Part model, mm, in its own coordinate system. Face numbers are marked on the shaded views. A direction names the side the tool comes from. Round coordinates to 2 decimals unless told otherwise and drop trailing zeros. Write each loop counter-clockwise with the first axis right and the second up, starting at its lowest first coordinate (ties: lowest second). Pieces come first, ordered by that corner, then holes. Notation, with made-up numbers: M -33.75,-22.75 L 16.25,-22.75 A12 cw 16.25,-2.75 Z; hole C 83,-34.75 d8. An arc over 180 degrees is marked long. Use a Markdown table: item, result. Add a question column.
1) Two-plate mould, pull along X, no slides. Class the marked faces 1, 2 and 3: released by +X, released by -X, zero draft, split by the parting line, or undercut.
2) Slice it at C-C on z = 5.5. Write the cut outline in (x, y), plus the area to 3 significant figures.
3) Which spindle directions (+Z, -Z, +X, -X, +Y, -Y) get a long thin tool onto all of the face, cutting with end or side? Do the marked faces 4 and 5. Say none if no direction does.
4) Slice it at D-D on y = 10. Write the cut outline in (x, z).
5) Slice it at B-B on y = -14.5. Write the cut outline in (x, z).
6) Slice it at A-A on z = 1.5. Write the cut outline in (x, y).
7) Wall check: probe 1 along Y at (x, z) = (3.25, 6.25); probe 2 along X at (y, z) = (-10, 1.25); probe 3 along X at (y, z) = (14.5, 3.75). Give the ranges that are in metal, low to high.
8) Drop flat-ended pins along their axis: P1, Ø4, axis at x = 1, y = 15, coming from the -Z side; P2, Ø0.5, axis at x = 8, z = 7, coming from the -Y side; P3, Ø2.5, axis at x = 6, y = -11, coming from the -Z side. Give the stop position or say it passes through.
Solid Edge part; units mm, degrees
sketch "Sketch1" plane through (0, 0, 0) normal (0, 0, 1) x (1, 0, 0)
  line L0 (-4, -20) -> (4, -20)
  line L1 (4, -20) -> (4, 20)
  line L2 (4, 20) -> (-4, 20)
  line L3 (-4, 20) -> (-4, -20)
  dimension "D1" = 4
  dimension "D2" = 4
extrude "Protrusion1" add sketch "Sketch1" along normal blind 10
sketch "Sketch2" plane through (0, 0, 10) normal (0, 0, 1) x (0, 1, 0)
  line L0 (-15.5, -4) -> (-17.5, -7.5)
  line L1 (-17.5, -7.5) -> (-17.5, -9)
  line L2 (-17.5, -9) -> (-7.5, -9)
  line L3 (-7.5, -9) -> (-7.5, -7.5)
  line L4 (-7.5, -7.5) -> (-9.5, -4)
  line L5 (-15.5, -4) -> (-9.5, -4)
  dimension "D1" = 17.5
  dimension "D2" = 15.5
  dimension "D3" = 7.5
  dimension "D4" = 17.5
extrude "Extrusionsausprägung_2" add sketch "Sketch2" against normal blind 8
chamfer "Fase_1" distance 0.5 angle 45 2 edges at (9, -17.5, 6) (9, -7.5, 6)
sketch "Sketch3" plane through (0, 0, 0) normal (0, 0, -1) x (0, 1, 0)
  line L0 (9.45, 4) -> (7, 0.55)
  line L1 (7, 0.55) -> (7, -1.05)
  line L2 (7, -1.05) -> (18, -1.05)
  line L3 (18, -1.05) -> (18, 0.55)
  line L4 (18, 0.55) -> (15.55, 4)
  line L5 (15.55, 4) -> (9.45, 4)
  dimension "D1" = 7
  dimension "D2" = 15.55
  dimension "D3" = 18
  dimension "D4" = 7
extrude "Extrusionsausschnitt_1" cut sketch "Sketch3" against normal blind 8.05
chamfer "Fase_2" distance 0.5 angle 45 2 edges at (-1.05, 18, 4.025) (-1.05, 7, 4.025)
fillet "Verrundung_1" radius 0.25 4 edges at (4, 15.55, 4.025) (4, 9.45, 4.025) (4, -9.5, 6) (4, -15.5, 6)
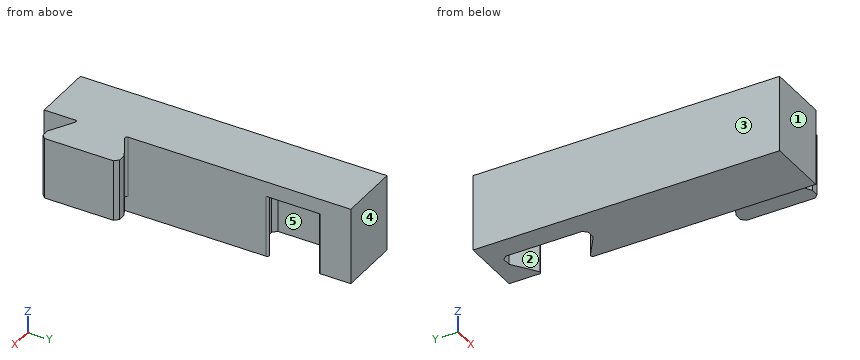
Entries:
| question | item | result |
|---|---|---|
| 1 | face 1 | zero draft |
| 1 | face 2 | undercut |
| 1 | face 3 | released by -X |
| 2 | outline | M -4,-20 L 4,-20 L 4,-15.93 A0.25 cw 4.37,-15.71 L 7.5,-17.5 L 8.5,-17.5 L 9,-17 L 9,-8 L 8.5,-7.5 L 7.5,-7.5 L 4.37,-9.29 A0.25 cw 4,-9.07 L 4,8.97 A0.25 ccw 3.61,9.17 L 0.55,7 L -0.55,7 L -1.05,7.5 L -1.05,17.5 L -0.55,18 L 0.55,18 L 3.61,15.83 A0.25 ccw 4,16.03 L 4,20 L -4,20 Z |
| 2 | area | 316 mm^2 |
| 3 | face 4 | +Z, -Z, +X, -X, +Y |
| 3 | face 5 | -Z |
| 4 | outline | M -4,0 L -1.05,0 L -1.05,8.05 L 4,8.05 L 4,10 L -4,10 Z |
| 5 | outline | M -4,0 L 4,0 L 4,2 L 9,2 L 9,10 L -4,10 Z |
| 6 | outline | M -4,-20 L 4,-20 L 4,8.97 A0.25 ccw 3.61,9.17 L 0.55,7 L -0.55,7 L -1.05,7.5 L -1.05,17.5 L -0.55,18 L 0.55,18 L 3.61,15.83 A0.25 ccw 4,16.03 L 4,20 L -4,20 Z |
| 7 | probe 1 | y = -20 to 8.92, 16.08 to 20 |
| 7 | probe 2 | x = -4 to 4 |
| 7 | probe 3 | x = -4 to -1.05 |
| 8 | P1 | stops at z = 8.05 |
| 8 | P2 | stops at y = -17.5 |
| 8 | P3 | stops at z = 2 |
